Input: part model. Units: mm. Frame: model coordinates. Face numbers are marked on the shaded views. Round coordinates to 2 decimals unless told otherwise and drop trailing zeros. Loops run counter-clockwise (first coordinate to the right, second up) from the corner with the lowest first, then second, coordinate; pieces in that order, holes last. Notation, with made-up numbers: M 28,68 L 87,68 A17 ccw 87,75 Z; hole C 29.5,-39 d6. An arc over 180 degrees is marked long. Return JSON: item names as keys, results as strings. Group by question number.
1) Section B-B (y = 0). Output: boundary loops of the cut face in (x, z), plus the area to 3 significant figures.
2) Contact query for flat-ended pins moving along their axis: P1, Ø4.5, axis at y = -1, z = 17, coming from the +X side; P2, Ø9, axis at x = -6.5, y = 5, coming from the -Z side; P3, Ø4.5, axis at x = 0, y = 0, coming from the +Z side. Output: stop coordinate, or through.
3) Section D-D (y = -22). Output: boundary loops of the cut face in (x, z).
4) Section C-C (z = 47). Output: boundary loops of the cut face in (x, y).
5) Section A-A (x = 0). Output: boundary loops of the cut face in (y, z), plus the area to 3 significant figures.
6) Material intervals for line 1 (X direction, y = 0, z = -48.75); line 2 (Y direction, x = 0, z = 13), sorted ascending. Write a range as from..to.
7) Mould query, pull axis Y, two halves, no side actions, for the marked faces 1, 2 and 3. Classes: +Y half, -Y half, draft (parallel to the pull), parting line (faces both ways), or undercut.
Autodesk Inventor part; units mm, degrees
ref_plane "YZ Plane" through (0, 0, 0) normal (1, 0, 0) x (0, 1, 0)
ref_plane "XZ Plane" through (0, 0, 0) normal (0, 1, 0) x (-1, 0, 0)
ref_plane "XY Plane" through (0, 0, 0) normal (0, 0, 1) x (1, 0, 0)
sketch "Sketch1" plane through (0, 0, 0) normal (0, 0, 1) x (1, 0, 0)
  circle A0 centre (0, 0) radius 37.5
  dimension "d0" = 75
extrude "Extrusion1" add sketch "Sketch1" along normal mid plane 110
sketch "Sketch5" plane through (0, 0, 55) normal (0, 0, 1) x (1, 0, 0)
  circle A0 centre (0, 0) radius 39
  dimension "d22" = 78
extrude "Extrusion4" add sketch "Sketch5" against normal blind 4
mirror "Mirror2" about plane through (0, 0, 0) normal (0, 0, 1) of "Extrusion4"
sketch "Sketch4" plane through (0, 0, -55) normal (0, 0, -1) x (-1, 0, 0)
  point P0 (0, 0)
  point P1 (0, 0)
hole "Hole1" at (0, 0, -55) direction (0, 0, 1) diameter 26 depth 40 counterbore diameter 30.2 counterbore depth 9.3
sketch "Sketch6" plane through (0, 0, 55) normal (0, 0, 1) x (1, 0, 0)
  circle A0 centre (0, 0) radius 2.55
  dimension "d25" = 5.1
extrude "Extrusion5" cut sketch "Sketch6" against normal blind 10
sketch "Sketch7" plane through (0, 0, 55) normal (0, 0, 1) x (1, 0, 0)
  circle A0 centre (0, 0) radius 2.55
  line L0 (-1.5, -2.0622) -> (-1.5, 2.0622)
  line L1 (1.5, 2.0622) -> (1.5, -2.0622)
  arc A1 (-1.5, -2.0622) -> (1.5, -2.0622) centre (0, 0) ccw
  arc A2 (1.5, 2.0622) -> (-1.5, 2.0622) centre (0, 0) ccw
  dimension "d28" = 1.5
extrude "Extrusion6" cut sketch "Sketch7" against normal through all contours L1 A0 L0
properties part number "13042026-14"
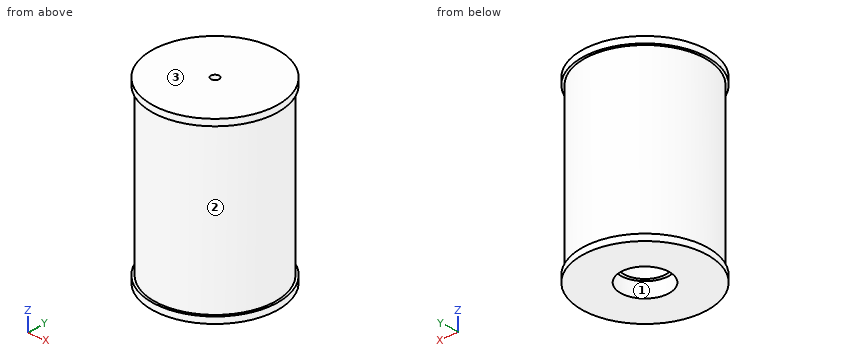
Returned:
{
 "1": {"outline": "M -39,-55 L -15.1,-55 L -15.1,-45.7 L -13,-45.7 L -13,-15 L -1.5,-15 L -1.5,45 L -2.55,45 L -2.55,55 L -39,55 L -39,51 L -37.5,51 L -37.5,-51 L -39,-51 Z; M 1.5,-15 L 13,-15 L 13,-45.7 L 15.1,-45.7 L 15.1,-55 L 39,-55 L 39,-51 L 37.5,-51 L 37.5,51 L 39,51 L 39,55 L 2.55,55 L 2.55,45 L 1.5,45 Z", "area": "6,960 mm^2"},
 "2": {"P1": "stops at x = 37.5", "P2": "stops at z = -15", "P3": "stops at z = 45"},
 "3": {"outline": "M -32.2,-55 L 32.2,-55 L 32.2,-51 L 30.37,-51 L 30.37,51 L 32.2,51 L 32.2,55 L -32.2,55 L -32.2,51 L -30.37,51 L -30.37,-51 L -32.2,-51 Z"},
 "4": {"outline": "C 0,0 d75; hole C 0,0 d5.1"},
 "5": {"outline": "M -39,-55 L -15.1,-55 L -15.1,-45.7 L -13,-45.7 L -13,-15 L -2.55,-15 L -2.55,55 L -39,55 L -39,51 L -37.5,51 L -37.5,-51 L -39,-51 Z; M 2.55,-15 L 13,-15 L 13,-45.7 L 15.1,-45.7 L 15.1,-55 L 39,-55 L 39,-51 L 37.5,-51 L 37.5,51 L 39,51 L 39,55 L 2.55,55 Z", "area": "6,840 mm^2"},
 "6": {"line 1": "x = -37.5..-15.1, 15.1..37.5", "line 2": "y = -37.5..-2.55, 2.55..37.5"},
 "7": {"face 1": "undercut", "face 2": "parting line", "face 3": "draft"}
}
